The drawing under review shows one solid part. Ordinate dimensions are in mm from its lowest x, y, z. A direction names the side the tool comes from. Round coordinates to 2 decimals unless told otherwise and drop trailing zeros. Write each loop counter-clockwise with the first axis right and the second up, starting at its lowest first coordinate (ties: lowest second). Pieces come first, ordered by that corner, then holes. Notation, with made-up numbers: (-34, 4) -> (-25, 4) arc R20 cw to (-25, 28) -> close; hole circle Ø4 at (75.5, 56.25). An arc over 180 degrees is marked (long way). Write item = value, one per line. Start each with the question number.
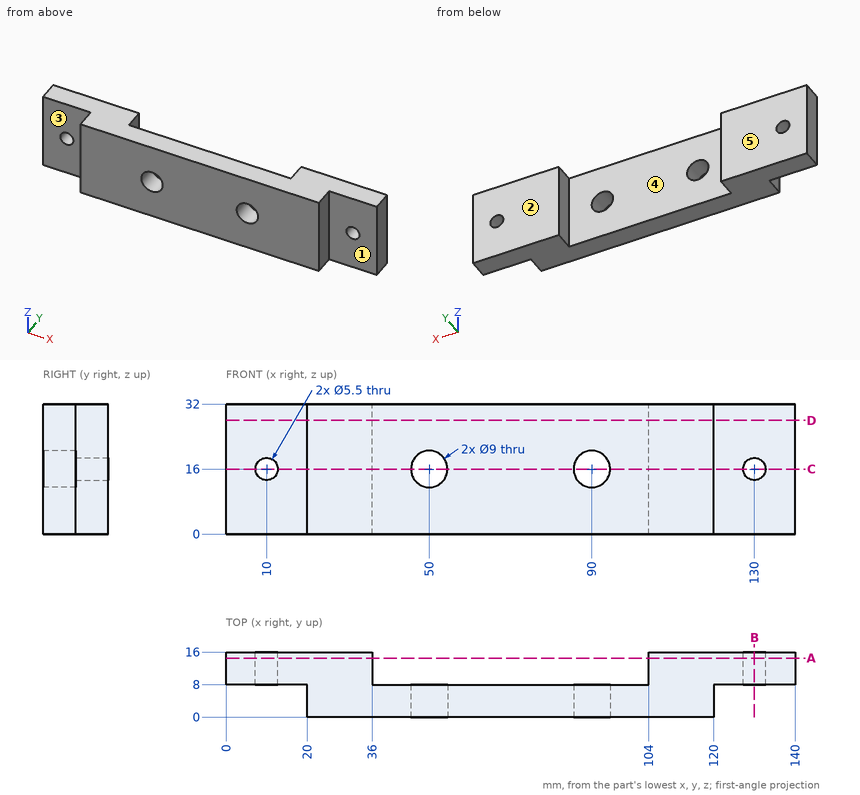
1. Consider section D-D, the plane z = 28. Give the boundary of the cut face in (x, y), then the cut area to 3 significant figures.
2. Consider section C-C, the plane z = 16. Give the boundary of the cut face in (x, y), then the cut area to 3 significant figures.
3. Machinability: for the marked faces 1, 2 and 3, which of the approach directions +Z, -Z, +X, -X, +Y, -Y give a long, thin tool a straight path to every point of the face, cutting with its end or side? Answer none if there is none.
4. Consider section A-A, the plane y = 14.5. Give the boundary of the cut face in (x, z), then the cut area to 3 significant figures.
5. Wall thickness on L1, parallel to X at y = 7.25, z = 15.5; L2, parallel to X at y = 13, z = 16; L3, parallel to X at y = 10.25, z = 27: over which ranges is each line inside the solid? List them lowest first. Write a range as from..to.
6. Draft analysis for pull direction X (two halves, no side actions). For the marked faces 4 and 5, state which applies: +X half, -X half, draft (parallel to the pull), parting line (faces both ways), or undercut.
7. Consider section B-B, the plane x = 130. Give the boundary of the cut face in (y, z).
8. Clearance check with flat-ended pins moving along their axes: pin 1 Ø3 at (x, z) = (16.5, 23.5) entering from -Y; pin 2 Ø2.5 at (y, z) = (2.5, 17) entering from +X; pin 3 Ø2 at (y, z) = (6.5, 17) entering from -X. State where each tip first meets the part, or that it passes through.
Outcome:
q1.outline = (0, 8) -> (20, 8) -> (20, 0) -> (120, 0) -> (120, 8) -> (140, 8) -> (140, 16) -> (104, 16) -> (104, 8) -> (36, 8) -> (36, 16) -> (0, 16) -> close
q1.area = 1,380 mm2
q2.outline = (0, 8) -> (7.25, 8) -> (7.25, 16) -> (0, 16) -> close; (12.75, 8) -> (20, 8) -> (20, 0) -> (45.5, 0) -> (45.5, 8) -> (36, 8) -> (36, 16) -> (12.75, 16) -> close; (54.5, 0) -> (85.5, 0) -> (85.5, 8) -> (54.5, 8) -> close; (94.5, 0) -> (120, 0) -> (120, 8) -> (127.25, 8) -> (127.25, 16) -> (104, 16) -> (104, 8) -> (94.5, 8) -> close; (132.75, 8) -> (140, 8) -> (140, 16) -> (132.75, 16) -> close
q2.area = 1,140 mm2
q3.face_1 = +Z, -Z, +X, -Y
q3.face_2 = +Z, -Z, +X, -X, +Y
q3.face_3 = +Z, -Z, -X, -Y
q4.outline = (0, 0) -> (36, 0) -> (36, 32) -> (0, 32) -> close; (104, 0) -> (140, 0) -> (140, 32) -> (104, 32) -> close; hole circle Ø5.5 at (10, 16); hole circle Ø5.5 at (130, 16)
q4.area = 2,260 mm2
q5.L1 = 20..45.53, 54.47..85.53, 94.47..120
q5.L2 = 0..7.25, 12.75..36, 104..127.25, 132.75..140
q5.L3 = 0..36, 104..140
q6.face_4 = undercut
q6.face_5 = draft
q7.outline = (8, 0) -> (16, 0) -> (16, 13.25) -> (8, 13.25) -> close; (8, 18.75) -> (16, 18.75) -> (16, 32) -> (8, 32) -> close
q8.pin_1 = 8
q8.pin_2 = 120
q8.pin_3 = 20
